The model under review builds one solid part; all positions refer to its coordinate system, in mm. Face numbers are marked on the shaded views. Give positions to 0.01 mm unless a question says otherwise; leave off trailing zeros. Return JSON: item names as keys, results as strings.
Autodesk Inventor part; units mm, degrees
ref_plane "YZ Plane" through (0, 0, 0) normal (1, 0, 0) x (0, 1, 0)
ref_plane "XZ Plane" through (0, 0, 0) normal (0, 1, 0) x (-1, 0, 0)
ref_plane "XY Plane" through (0, 0, 0) normal (0, 0, 1) x (1, 0, 0)
sketch "スケッチ1" plane through (0, 0, 0) normal (0, 0, 1) x (1, 0, 0)
  line L0 (108, 72.831817) -> (108, -27.637331) construction
  circle A0 centre (90, 27) radius 3
  circle A1 centre (104.07345, 2) radius 6.025
  circle A2 centre (90, 27) radius 1.5
  circle A3 centre (104.07345, 2) radius 1.5
  circle A4 centre (82.04031, 11.281864) radius 1.5
  circle A5 centre (82.5, -8) radius 3
  circle A6 centre (82.5, -8) radius 1.5
  arc A7 (66.645247, -5.64) -> (72.915941, -4.36) centre (69.780594, -5) ccw
  arc A8 (72.724551, 23.828571) -> (66.645247, -5.64) centre (104.07345, 2) ccw
  arc A9 (77.976723, 20.171429) -> (72.915941, -4.36) centre (104.07345, 2) ccw
  arc A10 (77.976723, 20.171429) -> (72.724551, 23.828571) centre (75.350637, 22) ccw
  circle A11 centre (137.322151, 20) radius 1.25
  circle A12 centre (133.5, -8) radius 3
  circle A13 centre (133.5, -8) radius 1.5
  circle A14 centre (146, 10) radius 1.5
  arc A15 (-6.089587, 13.373015) -> (73.990447, 1.93301) centre (42.288654, 66.020578) ccw construction
  line L1 (108, 72.831817) -> (108, -27.637331) construction
  arc A16 (142.009553, 1.93301) -> (222.089587, 13.373015) centre (173.711346, 66.020578) ccw construction
  arc A17 (142.29705, -19.072921) -> (142.660887, 27.253552) centre (125.709293, 4.222021) ccw
  arc A18 (136.80781, 35.127338) -> (180.06622, 10.718677) centre (180.861669, 62.665248) ccw
  circle A19 centre (137.322151, 20) radius 9.006449
  arc A20 (128.322651, 20.353731) -> (130.555913, -8.5765) centre (253.226204, 15.444317) ccw
  arc A21 (133.414591, -10.998784) -> (152.948723, -4.485529) centre (134.268683, 18.989056) ccw
  arc A22 (35.93378, 10.718677) -> (79.19219, 35.127338) centre (35.138331, 62.665248) ccw
  arc A23 (73.339113, 27.253552) -> (73.70295, -19.072921) centre (90.290707, 4.222021) ccw
  arc A24 (90.887703, 29.865656) -> (71.118535, 25.188537) centre (84.969685, 10.761283) ccw
  arc A25 (109.559222, 4.491371) -> (92.075879, 29.165808) centre (36.719095, -28.589074) ccw
  arc A26 (80.567193, -10.294397) -> (70.653319, -16.566942) centre (76.603177, -15) ccw
  circle A27 centre (76.603177, -15) radius 5 construction
  circle A28 centre (94, -11) radius 1.5
  circle A29 centre (94, -11) radius 3
  arc A30 (103.111347, -3.947687) -> (84.657245, -10.084777) centre (99.757959, -24.678215) ccw
  line L2 (108, 72.831817) -> (108, -27.637331) construction
  circle A31 centre (90, 27) radius 3
  circle A32 centre (104.07345, 2) radius 6.025
  circle A33 centre (90, 27) radius 1.5
  circle A34 centre (104.07345, 2) radius 1.5
  circle A35 centre (82.04031, 11.281864) radius 1.5
  circle A36 centre (82.5, -8) radius 3
  circle A37 centre (82.5, -8) radius 1.5
  arc A38 (66.645247, -5.64) -> (72.915941, -4.36) centre (69.780594, -5) ccw
  arc A39 (72.724551, 23.828571) -> (66.645247, -5.64) centre (104.07345, 2) ccw
  arc A40 (77.976723, 20.171429) -> (72.915941, -4.36) centre (104.07345, 2) ccw
  arc A41 (77.976723, 20.171429) -> (72.724551, 23.828571) centre (75.350637, 22) ccw
  circle A42 centre (137.322151, 20) radius 1.25
  circle A43 centre (133.5, -8) radius 4
  circle A44 centre (133.5, -8) radius 1.5
  circle A45 centre (146, 10) radius 1.5
  arc A46 (-6.089587, 13.373015) -> (73.990447, 1.93301) centre (42.288654, 66.020578) ccw construction
  line L3 (108, 72.831817) -> (108, -27.637331) construction
  arc A47 (142.009553, 1.93301) -> (222.089587, 13.373015) centre (173.711346, 66.020578) ccw construction
  arc A48 (142.29705, -19.072921) -> (142.660887, 27.253552) centre (125.709293, 4.222021) ccw
  arc A49 (136.80781, 35.127338) -> (180.06622, 10.718677) centre (180.861669, 62.665248) ccw
  circle A50 centre (137.322151, 20) radius 9.006449
  arc A51 (128.342019, 20.688016) -> (129.550355, -8.632697) centre (252.976757, 11.139082) ccw
  arc A52 (133.563777, -11.999492) -> (152.948723, -4.485529) centre (133.08545, 17.996695) ccw
  arc A53 (35.93378, 10.718677) -> (79.19219, 35.127338) centre (35.138331, 62.665248) ccw
  arc A54 (73.339113, 27.253552) -> (73.70295, -19.072921) centre (90.290707, 4.222021) ccw
  arc A55 (90.887703, 29.865656) -> (71.118535, 25.188537) centre (84.969685, 10.761283) ccw
  arc A56 (109.559222, 4.491371) -> (92.075879, 29.165808) centre (36.719095, -28.589074) ccw
  arc A57 (80.567193, -10.294397) -> (70.653319, -16.566942) centre (76.603177, -15) ccw
  circle A58 centre (76.603177, -15) radius 5 construction
  circle A59 centre (94, -11) radius 1.5
  circle A60 centre (94, -11) radius 3
  arc A61 (103.111347, -3.947687) -> (84.657245, -10.084777) centre (99.757959, -24.678215) ccw
  circle A62 centre (137.322151, 20) radius 1.5
  point P0 (0, 0)
  point P1 (0, 0)
  point P2 (0, 0)
  point P3 (153.490711, -2.560367)
  point P4 (70.420594, -8.135347)
  point P5 (68.814065, 23.104865)
  point P6 (143.754929, 26.303609)
  point P7 (147.185935, 23.104865)
  point P8 (0, 0)
  point P9 (153.490711, -2.560367)
  point P10 (152.948723, -4.485529)
  dimension "d0" = 2
  dimension "d1" = 30
  dimension "d2" = 125
  dimension "d3" = 80
  dimension "d4" = 20
  dimension "d5" = 6
  dimension "d6" = 21
  dimension "d14" = 2
  dimension "d15" = 30
  dimension "d16" = 125
  dimension "d17" = 80
  dimension "d18" = 20
  dimension "d19" = 6
  dimension "d20" = 21
  dimension "d25" = 3
extrude "押し出し1" add sketch "スケッチ1" along normal blind 3 contours A12 | A12 A20 A43 A21 | A12 A21 A43 A20 | A43 A51 A19 A20 | A20 A19 A18 A17 A21 A43 | A21 A52 A43 | A19
fillet "フィレット1" radius 3 1 edges at (152.9487, -4.4855, 1.5)
fillet "フィレット2" radius 5 1 edges at (147.1859, 23.1049, 1.5)
sketch "スケッチ3" plane through (0, 0, 0) normal (0, 0, -1) x (-1, 0, 0)
  arc A0 (-146.917757, 23.334729) -> (-147.45257, 22.797215) centre (-143.650945, 19.549502) ccw
  arc A1 (-147.45257, 22.797215) -> (-153.216482, -3.598627) centre (-125.709293, 4.222021) ccw
  arc A2 (-152.246999, -5.086525) -> (-133.563777, -11.999492) centre (-133.08545, 17.996695) ccw
  arc A3 (-133.563777, -11.999492) -> (-129.550355, -8.632697) centre (-133.5, -8) ccw
  arc A4 (-129.550355, -8.632697) -> (-128.342019, 20.688016) centre (-252.976757, 11.139082) ccw
  arc A5 (-128.342019, 20.688016) -> (-143.754929, 26.303609) centre (-137.322151, 20) ccw
  arc A6 (-146.917757, 23.334729) -> (-143.754929, 26.303609) centre (-180.861669, 62.665248) ccw
  circle A7 centre (-133.5, -8) radius 1.5
  circle A8 centre (-146, 10) radius 1.5
  circle A9 centre (-137.322151, 20) radius 3.1
  circle A10 centre (-146, 10) radius 3.1
  circle A11 centre (-133.5, -8) radius 3.1
  arc A12 (-153.216482, -3.598627) -> (-152.246999, -5.086525) centre (-150.330844, -2.778203) ccw
  circle A13 centre (-137.322151, 20) radius 1.5
  point P0 (0, 0)
  dimension "d21" = 6.2
  dimension "d22" = 6.2
  dimension "d23" = 6.2
extrude "押し出し2" cut sketch "スケッチ3" against normal blind 1 contours A9 | A10 | A11
sketch "スケッチ4" plane through (0, 0, 3) normal (0, 0, 1) x (1, 0, 0)
  arc A0 (147.45257, 22.797215) -> (146.917757, 23.334729) centre (143.650945, 19.549502) ccw
  arc A1 (143.754929, 26.303609) -> (146.917757, 23.334729) centre (180.861669, 62.665248) ccw
  arc A2 (143.754929, 26.303609) -> (128.342019, 20.688016) centre (137.322151, 20) ccw
  arc A3 (128.342019, 20.688016) -> (129.550355, -8.632697) centre (252.976757, 11.139082) ccw
  arc A4 (129.550355, -8.632697) -> (133.563777, -11.999492) centre (133.5, -8) ccw
  arc A5 (133.563777, -11.999492) -> (152.246999, -5.086525) centre (133.08545, 17.996695) ccw
  arc A6 (152.246999, -5.086525) -> (153.216482, -3.598627) centre (150.330844, -2.778203) ccw
  arc A7 (153.216482, -3.598627) -> (147.45257, 22.797215) centre (125.709293, 4.222021) ccw
  circle A8 centre (146, 10) radius 1.5
  circle A9 centre (137.322151, 20) radius 1.5
  circle A10 centre (133.5, -8) radius 1.5
  arc A11 (153.216482, -3.598627) -> (147.45257, 22.797215) centre (125.709293, 4.222021) ccw
  arc A12 (143.754929, 26.303609) -> (128.342019, 20.688016) centre (137.322151, 20) ccw
  spline S0 degree 2 poles (140.758179, 28.325252) (151.754441, 15.122285) (152.532068, -5.69497) knots 0 0 0 1 1 1
  circle A13 centre (146, 10) radius 3.1
  point P0 (0, 0)
  point P1 (148.894459, 14.077022)
  point P2 (140.758179, 28.325252)
  point P3 (153.361481, -3.069376)
  point P4 (152.496355, -4.854392)
  dimension "d36" = 5
  dimension "d37" = 13
  dimension "d38" = 17
  dimension "d39" = 36
extrude "押し出し3" cut sketch "スケッチ4" against normal blind 10 contours A7 A6 S0 A2 A1 A0
fillet "フィレット3" radius 10 1 edges at (152.4964, -4.8544, 1.5)
fillet "フィレット4" radius 5 1 edges at (140.7582, 28.3253, 1.5)
properties part number "アンノーン後" material "アルミニウム 2014-T4"
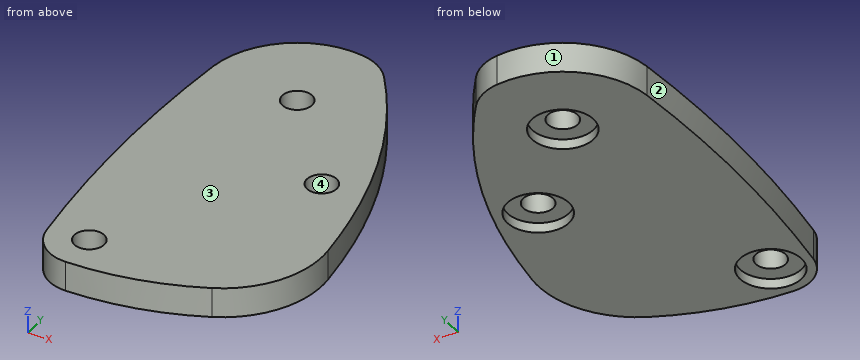
1) Consider section A-A on z = 1.75. Count the separate pieces of the cut face and the enclosed holes in it, then the cut area to 3 significant figures.
From the geometry:
{"separate pieces": "1", "enclosed holes": "3", "area": "758 mm²"}
2) The part is to be moulded in two halves that separate along Y. For the marked faces 1, 2, 3 and 4, say which applies: released by +Y, released by -Y, zero draft, split by the parting line, or undercut.
From the geometry:
{"face 1": "released by +Y", "face 2": "split by the parting line", "face 3": "zero draft", "face 4": "undercut"}
3) Insertion check: pin 1 (3 mm diameter, centred on x = 132.5, y = -9, fed in from -Z); pin 2 (1 mm diameter, centred on y = 12.5, z = 0.5, fed in from -X); pin 3 (1 mm diameter, centred on x = 144.5, z = 1.5, fed in from +Y). Each pin has a flat end and moves straight along its axis. Give the tip position at first contact, or say it passes through.
From the geometry:
{"pin 1": "z = 1", "pin 2": "x = 127.98", "pin 3": "y = 23.93"}
4) Wall thickness on L1, parallel to Y at x = 146, z = 1.85; L2, parallel to Y at x = 134, z = 1.4; L3, parallel to X at y = 19.5, z = 1.1: over which ranges is each line inside the solid? List them lowest first. Write a range as from..to.
From the geometry:
{"L1": "-9.08..8.5, 11.5..20.55", "L2": "-11.99..-9.41, -6.59..28.37", "L3": "128.26..135.91, 138.74..146.55"}
